Autodesk Inventor part; units mm, degrees
ref_plane "YZ Plane" through (0, 0, 0) normal (1, 0, 0) x (0, 1, 0)
ref_plane "XZ Plane" through (0, 0, 0) normal (0, 1, 0) x (-1, 0, 0)
ref_plane "XY Plane" through (0, 0, 0) normal (0, 0, 1) x (1, 0, 0)
sketch "Sketch1" plane through (0, 0, 0) normal (0, 1, 0) x (-1, 0, 0)
  line L0 (27.0344, 35.8723) -> (-27.9656, 35.8723)
  line L1 (27.0344, 35.8723) -> (27.0344, -39.1277)
  line L2 (27.0344, -39.1277) -> (-27.9656, -39.1277)
  line L3 (-27.9656, -39.1277) -> (-27.9656, 35.8723)
  line L4 (24.5344, 33.3723) -> (22.0344, 33.3723)
  line L5 (-25.4656, -36.6277) -> (-22.9656, -36.6277)
  line L6 (-25.4656, -36.6277) -> (-25.4656, -34.1277)
  line L7 (24.5344, -36.6277) -> (22.0344, -36.6277)
  line L8 (24.5344, -36.6277) -> (24.5344, -34.1277)
  line L9 (24.5344, 30.8723) -> (24.5344, 33.3723)
  line L10 (22.0344, 33.3723) -> (19.5344, 33.3723)
  line L11 (24.5344, 30.8723) -> (24.5344, 28.3723)
  line L12 (24.5344, 28.3723) -> (19.5344, 28.3723)
  line L13 (19.5344, 28.3723) -> (19.5344, 33.3723)
  line L14 (-20.4656, 33.3723) -> (-20.4656, 28.3723)
  line L15 (-20.4656, 28.3723) -> (-25.4656, 28.3723)
  line L16 (22.0344, -36.6277) -> (19.5344, -36.6277)
  line L17 (19.5344, -36.6277) -> (19.5344, -31.6277)
  line L18 (19.5344, -31.6277) -> (24.5344, -31.6277)
  line L19 (24.5344, -31.6277) -> (24.5344, -34.1277)
  line L20 (-22.9656, -36.6277) -> (-20.4656, -36.6277)
  line L21 (-20.4656, -36.6277) -> (-20.4656, -31.6277)
  line L22 (-20.4656, -31.6277) -> (-25.4656, -31.6277)
  line L23 (-25.4656, -31.6277) -> (-25.4656, -34.1277)
  line L24 (-30.4656, -41.6277) -> (-30.4656, 38.3723)
  line L25 (-30.4656, -41.6277) -> (29.5344, -41.6277)
  line L26 (29.5344, -41.6277) -> (29.5344, 38.3723)
  line L27 (29.5344, 38.3723) -> (-30.4656, 38.3723)
  line L28 (-20.4656, 33.3723) -> (-25.4656, 33.3723)
  line L29 (-25.4656, 33.3723) -> (-25.4656, 28.3723)
  point P0 (0, 0)
  dimension "d1" = 55
  dimension "d2" = 75
  dimension "d34" = 80
  dimension "d35" = 60
  dimension "d36" = 5
extrude "Extrusion1" add sketch "Sketch1" along normal blind 2 contours L1 L2 L3 L0
extrude "Extrusion2" add sketch "Sketch1" along normal blind 7 contours L9 L11 L12 L13 L10 L4 | L6 L23 L22 L21 L20 L5 | L7 L16 L17 L18 L19 L8 | L14 L15 L29 L28
extrude "Extrusion3" add sketch "Sketch1" along normal blind 20 contours L24 L27 L26 L25
sketch "Sketch2" plane through (-29.5344, 0, 38.3723) normal (0, 0, 1) x (1, 0, 0)
  line L0 (55, 7) -> (50, 7)
  line L1 (52.5, 7) -> (52.5, 8.5)
  line L2 (10, 7) -> (5, 7)
  line L3 (5, 7) -> (5, 8.5)
  line L4 (29.5344, 8.5) -> (37.0344, 8.5)
  line L5 (37.0344, 8.5) -> (37.0344, 16.5)
  line L6 (37.0344, 16.5) -> (22.0344, 16.5)
  line L7 (22.0344, 16.5) -> (22.0344, 8.5)
  line L8 (22.0344, 8.5) -> (29.5344, 8.5)
  point P0 (29.5344, 0)
  dimension "d43" = 1.5
extrude "Extrusion4" cut sketch "Sketch2" against normal blind 10
sketch "Sketch3" plane through (0, 2, 0) normal (0, 1, 0) x (1, 0, 0)
  line L0 (-24.5344, 36.6277) -> (-19.5344, 36.6277)
  line L1 (-17.0344, 36.6277) -> (-17.0344, 39.1277)
  line L2 (27.9656, 39.1277) -> (-27.0344, 39.1277)
  line L3 (-17.0344, 39.1277) -> (-27.0344, 39.1277)
  line L4 (-24.5344, 29.1277) -> (-27.0344, 29.1277)
  line L5 (-27.0344, 39.1277) -> (-27.0344, -35.8723)
  line L6 (-27.0344, 29.1277) -> (-27.0344, 39.1277)
  line L7 (-24.5344, 36.6277) -> (-24.5344, 31.6277)
  line L8 (-17.0344, 36.6277) -> (-24.5344, 36.6277)
  line L9 (-24.5344, 36.6277) -> (-24.5344, 29.1277)
  line L10 (27.9656, 39.1277) -> (17.9656, 39.1277)
  line L11 (27.9656, 39.1277) -> (27.9656, 29.1277)
  line L12 (27.9656, -35.8723) -> (27.9656, 39.1277)
  line L13 (17.9656, 39.1277) -> (17.9656, 36.6277)
  line L14 (25.4656, 36.6277) -> (20.4656, 36.6277)
  line L15 (17.9656, 36.6277) -> (25.4656, 36.6277)
  line L16 (25.4656, 36.6277) -> (25.4656, 29.1277)
  line L17 (25.4656, 29.1277) -> (27.9656, 29.1277)
  line L18 (-27.0344, -35.8723) -> (27.9656, -35.8723)
  line L19 (27.9656, -35.8723) -> (27.9656, -25.8723)
  line L20 (27.9656, -35.8723) -> (17.9656, -35.8723)
  line L21 (20.4656, -33.3723) -> (25.4656, -33.3723)
  line L22 (27.9656, -25.8723) -> (25.4656, -25.8723)
  line L23 (25.4656, -28.3723) -> (25.4656, -33.3723)
  line L24 (25.4656, -25.8723) -> (25.4656, -33.3723)
  line L25 (17.9656, -35.8723) -> (17.9656, -33.3723)
  line L26 (25.4656, -33.3723) -> (20.4656, -33.3723)
  line L27 (17.9656, -33.3723) -> (25.4656, -33.3723)
  line L28 (-27.0344, -35.8723) -> (-27.0344, -25.8723)
  line L29 (-27.0344, -35.8723) -> (-17.0344, -35.8723)
  line L30 (-17.0344, -35.8723) -> (-17.0344, -33.3723)
  line L31 (-17.0344, -33.3723) -> (-24.5344, -33.3723)
  line L32 (-24.5344, -33.3723) -> (-24.5344, -25.8723)
  line L33 (-24.5344, -25.8723) -> (-27.0344, -25.8723)
  point P0 (0, 0)
extrude "Extrusion5" add sketch "Sketch3" along normal blind 8 contours L7 L9 L4 L5 L2 L1 L8 L0
extrude "Extrusion6" add sketch "Sketch3" along normal blind 8 contours L2 L11 L17 L16 L14 L15 L13
extrude "Extrusion7" add sketch "Sketch3" along normal blind 8 contours L12 L18 L25 L27 L21 L23 L24 L22
extrude "Extrusion8" add sketch "Sketch3" along normal blind 8 contours L33 L32 L31 L30 L18 L5
sketch "Sketch4" plane through (-29.5344, 0, -41.6277) normal (-1, 0, 0) x (0, 0, 1)
  line L0 (0, 0) -> (0, 20)
  line L1 (17.5, 8.5) -> (17.5, 16.5)
  line L2 (17.5, 16.5) -> (32.5, 16.5)
  line L3 (32.5, 16.5) -> (32.5, 8.5)
  line L4 (17.5, 8.5) -> (32.5, 8.5)
  point P0 (41.6277, 0)
extrude "Extrusion9" cut sketch "Sketch4" against normal blind 5
properties part number "Caixa"
The model under review builds one solid part; all positions refer to its coordinate system, in mm. A direction names the side the tool comes from. Round coordinates to 2 decimals unless told otherwise and drop trailing zeros. Loops run counter-clockwise (first coordinate to the right, second up) from the corner with the lowest first, then second, coordinate; pieces in that order, holes last. Notation, with made-up numbers: M 77.25,50.5 L 120.25,50.5 A21 cw 120.25,54.5 Z; hole C 33.25,55.25 d7. An arc over 180 degrees is marked long. Put each result on its own line as item: value.
Q1. To check wall thickness, follow L1, parallel to Z at x = 7, y = 8; L2, parallel to Z at x = 25, y = 7.5; L3, parallel to X at y = 16, z = 0.5. State the ranges of each line that lie inside material, in increasing order.
Result set:
L1: z = -41.63 to -39.13, 35.87 to 38.37
L2: z = -41.63 to -36.63, 33.37 to 38.37
L3: x = -29.53 to -27.03, 27.97 to 30.47
Q2. Consider section D-D, the plane x = 19. Give the boundary of the cut face in (y, z), then the cut area to 3 significant figures.
Result set:
outline: M 0,-41.63 L 20,-41.63 L 20,-39.13 L 10,-39.13 L 10,-36.63 L 2,-36.63 L 2,33.37 L 10,33.37 L 10,35.87 L 20,35.87 L 20,38.37 L 0,38.37 Z
area: 290 mm²
Q3. Mouldability with a two-part tool opening along X and no side actions: class faces 1 (the flat face through (-24.534, 7, -31)), 2 (the flat face through (30.466, 10, -2)), 3 (the flat face through (-28, 12, -24.128)), 4 (the flat face through (20, 7, -36.628)) as released by +X, released by -X, zero draft, split by the parting line, or undercut.
Result set:
face 1: undercut
face 2: released by +X
face 3: zero draft
face 4: undercut
Q4. Consider section A-A, the plane x = 4.5. Give the boundary of the cut face in (y, z).
Result set:
outline: M 0,-41.63 L 20,-41.63 L 20,-39.13 L 2,-39.13 L 2,35.87 L 8.5,35.87 L 8.5,38.37 L 0,38.37 Z; M 16.5,35.87 L 20,35.87 L 20,38.37 L 16.5,38.37 Z
Q5. Machinability: for faces 5 (the flat face through (0, 16.5, 37)), 6 (the flat face through (20.466, 4, -34)), which of the approach directions +Z, -Z, +X, -X, +Y, -Y give a long, thin tool a straight path to every point of the face, cutting with its end or side? Answer none if there is none.
Result set:
face 5: +Z
face 6: +Y
Q6. Consider section B-B, the plane y = 18. Give the boundary of the cut face in (x, z).
Result set:
outline: M -29.53,-41.63 L 30.47,-41.63 L 30.47,38.37 L -29.53,38.37 Z; hole M -27.03,-39.13 L 27.97,-39.13 L 27.97,35.87 L -27.03,35.87 Z
Q7. Consider section C-C, the plane z = -14. Give the boundary of the cut face in (x, y).
Result set:
outline: M -29.53,0 L 30.47,0 L 30.47,20 L 27.97,20 L 27.97,2 L -27.03,2 L -27.03,8.5 L -29.53,8.5 Z; M -29.53,16.5 L -27.03,16.5 L -27.03,20 L -29.53,20 Z
Q8. For pin 1 (3 mm diameter, centred on x = 22, z = -35, fed in from +Y); pin 2 (1 mm diameter, centred on x = -11, z = 15, fed in from +Y), all flat-tipped, find the tip position at first contact; note any pin that passes through.
Result set:
pin 1: stops at y = 7
pin 2: stops at y = 2
